Could you check a few things on this model? Use its own coordinates, in mm. Face numbers are marked on the shaded views. Round coordinates to 2 decimals unless told otherwise and drop trailing zeros. Order: outer loops, then holes, each group sorted by start corner. A loop starts at its lowest first (then second) coordinate and runs counter-clockwise, first axis right, second up. Notation, with made-up numbers: (44, 70) - (63, 70) arc R21 ccw to (63, 80) - close; hole circle Ø5 at (25, 22). An arc over 180 degrees is marked (long way). Use one line per item in the form item = value.
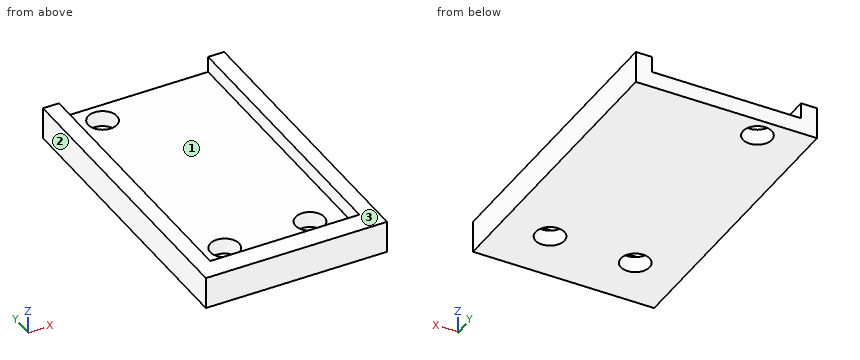
Autodesk Inventor part; units mm, degrees
ref_plane "YZ Plane" through (0, 0, 0) normal (1, 0, 0) x (0, 1, 0)
ref_plane "XZ Plane" through (0, 0, 0) normal (0, 1, 0) x (-1, 0, 0)
ref_plane "XY Plane" through (0, 0, 0) normal (0, 0, 1) x (1, 0, 0)
sketch "Sketch1" plane through (0, 0, 0) normal (0, 0, 1) x (1, 0, 0)
  line L0 (-17, 28) -> (0, 28)
  line L1 (0, 7) -> (0, 0)
  line L2 (0, 0) -> (-17, 0)
  line L3 (-17, 0) -> (-17, 7)
  line L4 (-17, 28) -> (-17, 17)
  line L5 (0, 28) -> (0, 17)
  line L6 (-17, 17) -> (-17, 7)
  line L7 (0, 17) -> (0, 7)
  point P0 (0, 0)
  point P1 (4, 7)
  point P2 (4, 7)
  dimension "d0" = 17
  dimension "d2" = 28
extrude "Extrusion1" add sketch "Sketch1" along normal blind 3
sketch "Sketch2" plane through (0, 0, 3) normal (0, 0, 1) x (1, 0, 0)
  line L0 (-17, 28) -> (-17, 0)
  line L1 (-17, 0) -> (0, 0)
  line L2 (0, 0) -> (0, 28)
  line L3 (0, 28) -> (-17, 28)
  line L4 (-17, 0) -> (0, 0)
  line L5 (-15.5, 2) -> (-1.5, 2)
  line L6 (-1.5, 2) -> (-1.5, 28)
  line L7 (-1.5, 28) -> (-15.5, 28)
  line L8 (-15.5, 28) -> (-15.5, 2)
  line L9 (0, 28) -> (-17, 28)
  dimension "d7" = 14
  dimension "d19" = 26
extrude "Extrusion2" cut sketch "Sketch2" against normal blind 1.5 contours L3 L6 L5 L8
sketch "Sketch3" plane through (0, 0, 1.5) normal (0, 0, 1) x (1, 0, 0)
  line L0 (-1.5, 28) -> (-1.5, 2)
  line L1 (-15.5, 28) -> (-1.5, 28)
  line L2 (-15.5, 2) -> (-15.5, 28)
  circle A0 centre (-12.5, 26) radius 1.35
  circle A1 centre (-12.5, 5) radius 1.35
  circle A2 centre (-4.5, 5) radius 1.35
  line L3 (-1.5, 2) -> (-15.5, 2)
  point P0 (0, 0)
  dimension "d12" = 2.7
  dimension "d13" = 8
  dimension "d14" = 21
  dimension "d21" = 3
extrude "Extrusion3" cut sketch "Sketch3" against normal through all contours A0 | A1 | A2
properties part number "soporte"
Item 1: I need wall thicknesses on L1, parallel to X at y = 14.25, z = 1.8; L2, parallel to Y at x = -12.5, z = 0.35; L3, parallel to Y at x = -4.5, z = 0.7. Which ranges of each line are inside material? Lowest first, please.
Found:
L1 = -17 to -15.5, -1.5 to 0
L2 = 0 to 3.65, 6.35 to 24.65, 27.35 to 28
L3 = 0 to 3.65, 6.35 to 28
Item 2: Imagine slicing it at A-A on x = -4.5. Please give me the cut outline in (y, z), plus the area to 4 significant figures.
Found:
outline = (0, 0) - (3.65, 0) - (3.65, 1.5) - (2, 1.5) - (2, 3) - (0, 3) - close; (6.35, 0) - (28, 0) - (28, 1.5) - (6.35, 1.5) - close
area = 40.95 mm2
Item 3: Imagine slicing it at C-C on z = 2.15. Please give me the cut outline in (x, y).
Found:
outline = (-17, 0) - (0, 0) - (0, 28) - (-1.5, 28) - (-1.5, 2) - (-15.5, 2) - (-15.5, 28) - (-17, 28) - close
Item 4: Imagine slicing it at D-D on x = -12.5. Please give me the cut outline in (y, z).
Found:
outline = (0, 0) - (3.65, 0) - (3.65, 1.5) - (2, 1.5) - (2, 3) - (0, 3) - close; (6.35, 0) - (24.65, 0) - (24.65, 1.5) - (6.35, 1.5) - close; (27.35, 0) - (28, 0) - (28, 1.5) - (27.35, 1.5) - close
Item 5: Will these pins go through, and if not, where does the flat tip stop? P1, Ø2.5, axis at x = -12.5, y = 5, coming from the +Z side; P2, Ø1.2, axis at x = -10.5, z = 2.5, coming from the +Y side; P3, Ø1, axis at x = -5.5, y = 18, coming from the +Z side.
Found:
P1 = through
P2 = 2
P3 = 1.5
Item 6: Imagine slicing it at B-B on y = 26. Please give me the cut outline in (x, z), plus the area to 4 significant figures.
Found:
outline = (-17, 0) - (-13.85, 0) - (-13.85, 1.5) - (-15.5, 1.5) - (-15.5, 3) - (-17, 3) - close; (-11.15, 0) - (0, 0) - (0, 3) - (-1.5, 3) - (-1.5, 1.5) - (-11.15, 1.5) - close
area = 25.95 mm2
Item 7: If we mould it in two halves opening along X, with no side actions, what happens to the marked faces 1, 2 and 3? For each: released by +X, released by -X, zero draft, split by the parting line, or undercut.
Found:
face_1 = undercut
face_2 = released by -X
face_3 = zero draft
